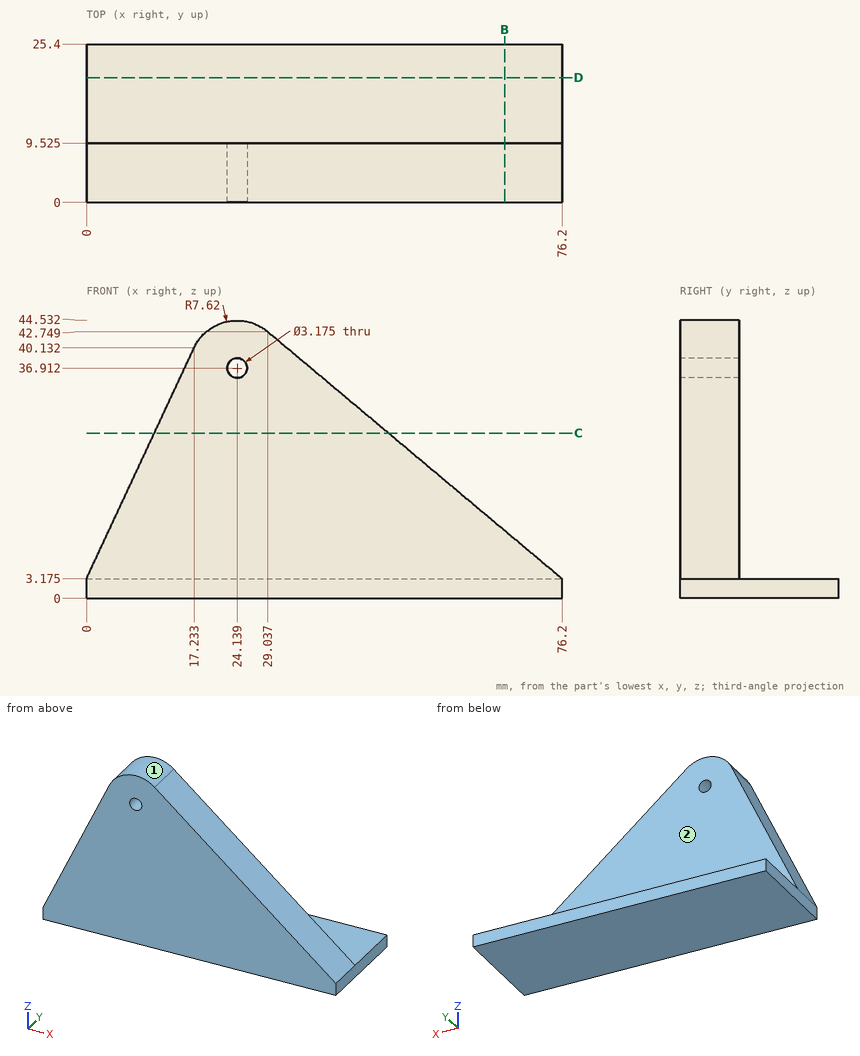
For this review, use the dimensioned drawing (mm, ordinates from the lowest corner) and the shaded views. A direction names the side the tool comes from. Round coordinates to 2 decimals unless told otherwise and drop trailing zeros. Order: outer loops, then holes, each group sorted by start corner. A loop starts at its lowest first (then second) coordinate and runs counter-clockwise, first axis right, second up. Notation, with made-up numbers: (-39, -14) -> (-15, -14) arc R23 cw to (-15, 20) -> close; hole circle Ø8 at (17, 40.25). An arc over 180 degrees is marked (long way). One line per item, written item: value. Start each with the question number.
Q1. Take a section at B-B (x = 67). Write out the cut boundary in (y, z) (1 decimal), and give its area (3 significant figures).
Q2. Take a section at C-C (z = 26.5). Write out the cut boundary in (x, y) (1 decimal).
Q3. Machinability: for the marked faces 1 and 2, which of the approach directions +Z, -Z, +X, -X, +Y, -Y give a long, thin tool a straight path to every point of the face, cutting with its end or side? Answer none if there is none.
Q4. Take a section at D-D (y = 20). Write out the cut boundary in (x, z) (1 decimal).
Q5. Wall thickness on line 1 (Z direction, x = 24.5, y = 24) (1 decimal); line 2 (Y direction, x = 53, z = 7.5) (1 decimal); line 3 (Z direction, x = 68, y = 8.75) (1 decimal): over which ranges is each line inside the solid? List them lowest first.
Q6. Clearance check with flat-ended pins moving along their axes: pin 1 Ø12.5 at (x, z) = (33, 31) entering from +Y (1 decimal); pin 2 Ø10 at (y, z) = (9.5, 12.5) entering from +X (1 decimal); pin 3 Ø12 at (y, z) = (11.5, 29.5) entering from -X. State where each tip first meets the part, or that it passes through.
Reported:
1. outline: (0, 0) -> (25.4, 0) -> (25.4, 3.2) -> (9.5, 3.2) -> (9.5, 10.9) -> (0, 10.9) -> close
1. area: 154 mm2
2. outline: (10.9, 0) -> (48.4, 0) -> (48.4, 9.5) -> (10.9, 9.5) -> close
3. face 1: +Z, +Y, -Y
3. face 2: +Z, +X, -X, +Y
4. outline: (0, 0) -> (76.2, 0) -> (76.2, 3.2) -> (0, 3.2) -> close
5. line 1: z = 0 to 3.2
5. line 2: y = 0 to 9.5
5. line 3: z = 0 to 10.1
6. pin 1: stops at y = 9.5
6. pin 2: stops at x = 71
6. pin 3: stops at x = 9.63
